Autodesk Fusion 360 part; units mm, degrees
sketch "Sketch1" plane through (0, 0, 0) normal (0, 0, 1) x (1, 0, 0)
  line L0 (28.5, -18) -> (-28.5, -18)
  line L1 (-28.5, -18) -> (-28.5, 18)
  line L2 (-28.5, 18) -> (28.5, 18)
  line L3 (28.5, 18) -> (28.5, -18)
  line L4 (28.5, -18) -> (-28.5, 18) construction
  line L5 (-28.5, -18) -> (28.5, 18) construction
  dimension "d1" = 57
  dimension "d2" = 36
extrude "Extrude1" add sketch "Sketch1" along normal blind 30
sketch "Sketch2" plane through (0, 0, 30) normal (0, 0, 1) x (-1, 0, 0)
  line L0 (-28.5, -18) -> (28.5, -18)
  line L1 (28.5, -18) -> (28.5, 18)
  line L2 (28.5, 18) -> (-28.5, 18)
  line L3 (-28.5, 18) -> (-28.5, -18)
  line L4 (28.5, 18) -> (28.5, 15)
  line L5 (-28.5, 15) -> (28.5, 15)
  line L6 (-28.5, 15) -> (-28.5, 18)
  line L7 (-28.5, 18) -> (28.5, 18)
  dimension "d7" = 3
extrude "Extrude2" add sketch "Sketch2" along normal blind 10 contours L1 L2 L3 L4 L5 L6 L7
mirror "Mirror1" about plane through (0, 0, 0) normal (0, 1, 0) of "Extrude2"
sketch "Sketch3" plane through (0, 0, 30) normal (0, 0, 1) x (-1, 0, 0)
  line L0 (-28.5, -15) -> (28.5, -15)
  line L1 (28.5, -15) -> (28.5, 15)
  line L2 (28.5, 15) -> (-28.5, 15)
  line L3 (-28.5, 15) -> (-28.5, -15)
  circle A0 centre (14.5, -2) radius 7.25
  dimension "d10" = 14.5
  dimension "d11" = 14
  dimension "d15" = 17
  dimension "d18" = 13
extrude "Extrude3" cut sketch "Sketch3" against normal through all contours A0
sketch "Sketch4" plane through (0, 0, 30) normal (0, 0, 1) x (-1, 0, 0)
  circle A0 centre (14.5, -2) radius 7.25
  line L0 (-28.5, -15) -> (28.5, -15)
  line L1 (28.5, -15) -> (28.5, 15)
  line L2 (28.5, 15) -> (-28.5, 15)
  line L3 (-28.5, 15) -> (-28.5, -15)
  line L4 (18.9159, -7.75) -> (28.5, -7.75)
  line L5 (28.5, -7.75) -> (28.5, 3.75)
  line L6 (18.9159, 3.75) -> (18.9159, -7.75)
  line L7 (18.9159, 3.75) -> (28.5, 3.75)
  dimension "d13" = 11.5
extrude "Extrude4" cut sketch "Sketch4" against normal through all contours A0 L1 L4 L5 L7
fillet "Fillet1" radius 2 2 edges at (0, -15, 30) (0, 15, 30)
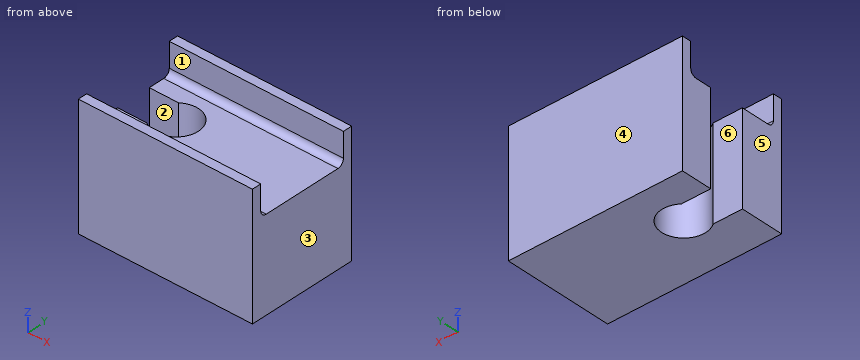
The model under review builds one solid part; all positions refer to its coordinate system, in mm. Face numbers are marked on the shaded views. A direction names the side the tool comes from. Coordinates: 2 decimals unless noted, no trailing zeros. Write each loop counter-clockwise with the first axis right and the second up, starting at its lowest first coordinate (ties: lowest second). Pieces come first, ordered by that corner, then holes. Notation, with made-up numbers: (36.5, 21) -> (74.5, 21) arc R23 cw to (74.5, 41) -> close; hole circle Ø8 at (-30.75, 46.25). An arc over 180 degrees is marked (long way). Answer in a Markdown table with one row per item.
1. We need section B-B, the plane z = 36. State the section outline as (x, y) points, and give its area (3 significant figures).
Answers below:
| item | result |
|---|---|
| outline | (-28.5, -18) -> (28.5, -18) -> (28.5, -15) -> (-28.5, -15) -> close; (-28.5, 15) -> (28.5, 15) -> (28.5, 18) -> (-28.5, 18) -> close |
| area | 342 mm^2 |
2. Draft analysis for pull direction Y (two halves, no side actions). For the marked faces 4, 5 and 6, state which applies: +Y half, -Y half, draft (parallel to the pull), parting line (faces both ways), or undercut.
Answers below:
| item | result |
|---|---|
| face 4 | +Y half |
| face 5 | draft |
| face 6 | undercut |
3. We need section D-D, the plane x = -6. State the section outline as (y, z) points, and give its area (3 significant figures).
Answers below:
| item | result |
|---|---|
| outline | (-18, 0) -> (18, 0) -> (18, 40) -> (15, 40) -> (15, 32) arc R2 cw to (13, 30) -> (-13, 30) arc R2 cw to (-15, 32) -> (-15, 40) -> (-18, 40) -> close |
| area | 1,140 mm^2 |
4. We need section C-C, the plane z = 9.5. State the section outline as (x, y) points.
Answers below:
| item | result |
|---|---|
| outline | (-28.5, -18) -> (28.5, -18) -> (28.5, 18) -> (-28.5, 18) -> (-28.5, 7.75) -> (-18.92, 7.75) arc R7.25 cw (long way) to (-18.92, -3.75) -> (-28.5, -3.75) -> close |
5. Clearance check with flat-ended pins moving along their axes: pin 1 Ø8 at (x, y) = (19.5, -8.5) entering from +Z; pin 2 Ø3 at (x, y) = (19, 13) entering from +Z. State where each tip first meets the part, or that it passes through.
Answers below:
| item | result |
|---|---|
| pin 1 | stops at z = 30 |
| pin 2 | stops at z = 30.68 |
6. Wall thickness on probe 1 along Y at (x, z) = (-14.5, 10.5); probe 2 along X at (y, z) = (2, 14); probe 3 along Y at (x, z) = (-18.5, 19.5): over which ranges is each line inside the solid? List them lowest first. Write a range as [from, to].
Answers below:
| item | result |
|---|---|
| probe 1 | y = [-18, -5.25], [9.25, 18] |
| probe 2 | x = [-7.25, 28.5] |
| probe 3 | y = [-18, -4.05], [8.05, 18] |
7. For the marked faces 1, 2 and 3, list the 3-axis set-ups (+Z, -Z, +X, -X, +Y, -Y) from which the entire face can be reached by the end or side of a thin tool; tool diameter is ignored.
Answers below:
| item | result |
|---|---|
| face 1 | +Z, +X, -X |
| face 2 | +Z, -Z, -X |
| face 3 | +Z, -Z, +X, +Y, -Y |
8. We need section A-A, the plane x = -14.5. State the section outline as (y, z) points, and give its area (3 significant figures).
Answers below:
| item | result |
|---|---|
| outline | (-18, 0) -> (-5.25, 0) -> (-5.25, 30) -> (-13, 30) arc R2 cw to (-15, 32) -> (-15, 40) -> (-18, 40) -> close; (9.25, 0) -> (18, 0) -> (18, 40) -> (15, 40) -> (15, 32) arc R2 cw to (13, 30) -> (9.25, 30) -> close |
| area | 707 mm^2 |
